Check sheet for the modelled part. Datum: model origin and axes. Units: mm. Give positions to 0.01 mm unless a question says otherwise; leave off trailing zeros. Order: outer loops, then holes, each group sorted by start corner. A loop starts at its lowest first (then second) coordinate and runs counter-clockwise, first axis right, second up. Notation, with made-up numbers: (57.5, 22.5) -> (113.5, 22.5) arc R20 ccw to (113.5, 40.5) -> close; hole circle Ø3 at (-28, 66). An arc over 180 degrees is marked (long way). Answer in a Markdown table with one row per item. Add a question column.
(1) Cross-section at A-A (z = 2). State how many separate pieces and enclosed holes the cut face has, then the cut area to 3 significant figures.
(2) Thickness scan on L1, parallel to X at y = 84, z = 0.55; L2, parallel to X at y = 14.5, z = 0.8; L3, parallel to Y at x = 41, z = 1.5. Record the ranges inside material, lowest first. Write a range as [from, to].
(3) Cross-section at B-B (x = 67.5). Record the cut outline in (y, z).
```python
from build123d import *

# Parameters (mm, degrees)
SKETCH1_W           = 145.885353282
SKETCH1_H           = 101.6
BOSS_EXTRUDE1_DEPTH = 3.2004
SKETCH4_W           = 57.100000132
SKETCH4_H           = 31.75
CUT_EXTRUDE1_DEPTH  = 3.2004
SKETCH5_R           = 2.159
CUT_EXTRUDE2_DEPTH  = 3.2004
FILLET1_R           = 0.762


with BuildPart() as part:
    # Sketch1 → Boss-Extrude1 (new body)
    with BuildSketch(Plane.XY):
        with Locations((72.942676641, 50.8)):
            Rectangle(SKETCH1_W, SKETCH1_H)
    extrude(amount=BOSS_EXTRUDE1_DEPTH)

    # Sketch4 → Cut-Extrude1 (cut)
    with BuildSketch(Plane.XY.offset(3.2004)):
        with Locations((56.982760066, 15.875)):
            Rectangle(SKETCH4_W, SKETCH4_H)
    extrude(amount=-CUT_EXTRUDE1_DEPTH, mode=Mode.SUBTRACT)

    # Sketch5 → Cut-Extrude2 (cut)
    with BuildSketch(Plane.XY.offset(3.2004)):
        with Locations((141.376853282, 82.55)):
            Circle(SKETCH5_R)
        with Locations((141.376853282, 19.05)):
            Circle(SKETCH5_R)
        with Locations((4.5085, 19.05)):
            Circle(SKETCH5_R)
        with Locations((4.5085, 82.55)):
            Circle(SKETCH5_R)
        with Locations((21.31994339, 79.375)):
            Circle(SKETCH5_R)
        with Locations((21.31994339, 22.225)):
            Circle(SKETCH5_R)
        with Locations((122.472903282, 79.375)):
            Circle(SKETCH5_R)
        with Locations((122.472903282, 22.225)):
            Circle(SKETCH5_R)
    extrude(amount=-CUT_EXTRUDE2_DEPTH, mode=Mode.SUBTRACT)

    # Fillet1
    fillet1_edges = [part.edges().sort_by_distance(p)[0] for p in [
        (28.43276, 0, 1.6002),
        (85.532760132, 0, 1.6002),
        (0, 101.6, 1.6002),
        (145.885353282, 101.6, 1.6002),
        (145.885353282, 0, 1.6002),
        (0, 0, 1.6002),
    ]]
    fillet(fillet1_edges, radius=FILLET1_R)


solid = part.part
```
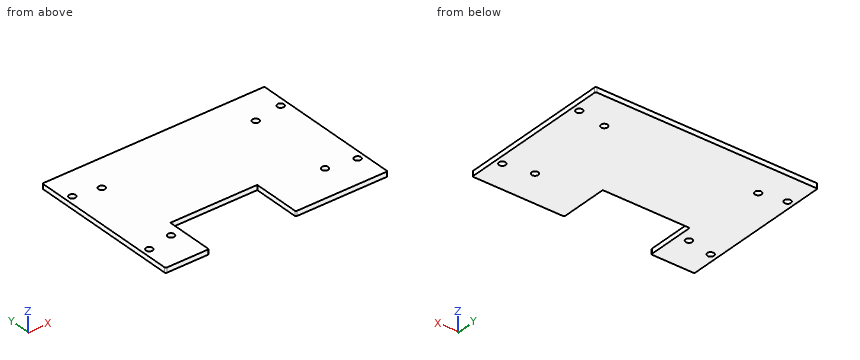
Answer below:
| question | item | result |
|---|---|---|
| 1 | separate pieces | 1 |
| 1 | enclosed holes | 8 |
| 1 | area | 12,900 mm² |
| 2 | L1 | x = [0, 2.91], [6.11, 139.78], [142.98, 145.89] |
| 2 | L2 | x = [0, 28.43], [85.53, 145.89] |
| 2 | L3 | y = [31.75, 101.6] |
| 3 | outline | (31.75, 0) -> (101.6, 0) -> (101.6, 3.2) -> (31.75, 3.2) -> close |
